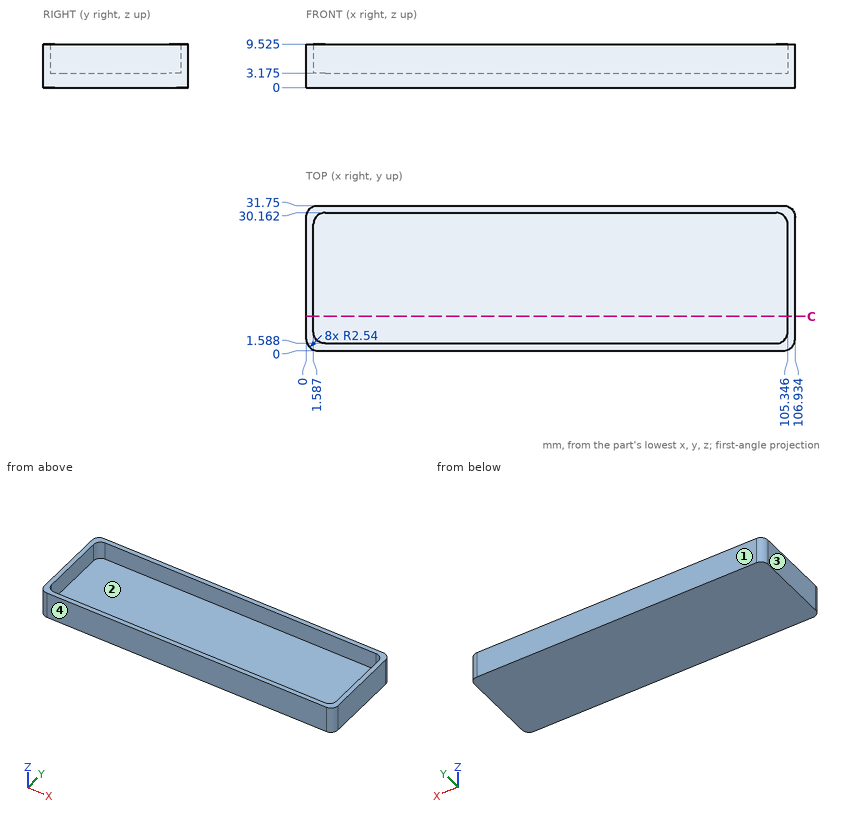
Study the drawing (mm; zero at the part's minimum x, y, z) and answer. Give positions to 0.01 mm unless a question says otherwise; leave off trailing zeros. Loops run counter-clockwise (first coordinate to the right, second up) from the corner with the lowest first, then second, coordinate; pieces in that order, holes last. Notation, with made-up numbers: (10.25, 13) - (28.25, 13) arc R14 cw to (28.25, 38) - close; hole circle Ø6 at (63.25, -9). An arc over 180 degrees is marked (long way). Return JSON: item names as keys, results as strings. Group by question number.
1. Straight lines are drawn through the part: line 1 (X direction, y = 5, z = 8.5) (1 decimal); line 2 (Y direction, x = 79, z = 9); line 3 (Z direction, x = 46.5, y = 24.5) (1 decimal). For each, find the intervals that lie inside material, in ascending order. Write a range as [from, to].
2. Determine the mould class of the marked faces 1, 2, 3 and 4 for opening direction Y: pulls with the +Y half, pulls with the -Y half, needs draft (parallel to the pull), parting line crosses it, or undercut.
3. Find section C-C (y = 7.5). Write down the section's boundary in (x, z) (1 decimal).
4. Given pin 1 Ø10 at (x, y) = (96, 8) entering from +Z (1 decimal), flat-ended and moving along its own axis, determine where the tip first touches the part or whether it passes through.
Verdict:
{
 "1": {"line 1": "x = [0, 1.6], [105.3, 106.9]", "line 2": "y = [0, 1.59], [30.16, 31.75]", "line 3": "z = [0, 3.2]"},
 "2": {"face 1": "pulls with the +Y half", "face 2": "undercut", "face 3": "needs draft", "face 4": "pulls with the -Y half"},
 "3": {"outline": "(0, 0) - (106.9, 0) - (106.9, 9.5) - (105.3, 9.5) - (105.3, 3.2) - (1.6, 3.2) - (1.6, 9.5) - (0, 9.5) - close"},
 "4": {"pin 1": "stops at z = 3.2"}
}
